The listing builds one solid part. Answer for the finished solid, in the listing's coordinates (mm). A direction names the side the tool comes from. Coordinates: 2 decimals unless noted, no trailing zeros. Order: outer loops, then holes, each group sorted by start corner. A loop starts at its lowest first (then second) coordinate and runs counter-clockwise, first axis right, second up. Notation, with made-up numbers: (9.5, 9.5) - (61.5, 9.5) arc R16 cw to (61.5, 37.5) - close; hole circle Ø2 at (74, 13). An arc over 180 degrees is marked (long way). Use a Markdown table: item, result. Add a question column.
Item 1: The part is cut by section C-C, the plane y = 3. Give the vertices of the cut face in (x, z).
Item 2: For faces 1 (the cylindrical face through (-17.572, 8.458, -3.902)), 2 (the flat face through (34, -20, 0)), determine the directions among +Z, -Z, +X, -X, +Y, -Y from which every point of the face is accessible in a straight line to the end or side of a thin tool.
Item 3: The part is cut by section D-D, the plane y = -6.5. Give the vertices of the cut face in (x, z), then the cut area to 3 significant figures.
Item 4: The part is cut by section A-A, the plane z = 0. Give the vertices of the cut face in (x, y), then the cut area to 3 significant figures.
Item 5: The part is cut by section B-B, the plane x = 0. Give the vertices of the cut face in (y, z).
Item 6: Flat-ended cylindrical pins translate along their axes: P1, Ø5, axis at y = -13, z = -0.5, coming from the +X side; P2, Ø12, axis at y = -0.5, z = 13.5, coming from the -X side; P3, Ø10, axis at x = -1, z = -2.5, coming from the +Y side; P4, Ø3, axis at y = 8.5, z = -5.5, coming from the +X side. Find the tip coordinate at first contact, or state that the pin passes through.
Item 7: Find the intervals of material crossed by line 1 along X through (y, z) = (4, 0); line 2 along X through (y, z) = (-5.75, 0); line 3 along Y through (x, z) = (30, 8), in increasing order.
from build123d import *

# Parameters (mm, degrees)
SKETCH1_R           = 18
BOSS_EXTRUDE1_DEPTH = 14
SKETCH2_R           = 3.25
BOSS_EXTRUDE2_DEPTH = 6
SKETCH3_R           = 10
SKETCH3_R_2         = 3.25
BOSS_EXTRUDE3_DEPTH = 20
CUT_EXTRUDE1_REACH  = 63.514
SKETCH4_R           = 10.75


with BuildPart() as part:
    # Sketch1 → Boss-Extrude1 (new body)
    with BuildSketch(Plane(origin=(0, 0, 0), x_dir=(1, 0, 0), z_dir=(0, 1, 0))):
        with Locations(Location((0, 0, 0), (0, 0, 270))):
            Circle(SKETCH1_R)
    extrude(amount=BOSS_EXTRUDE1_DEPTH)

    # Sketch2 → Boss-Extrude2 (add)
    with BuildSketch(Plane.XZ):
        with BuildLine():
            Line((40.105263158, 9.775881906), (3.789473684, 17.59658743))
            ThreePointArc((3.789473684, 17.59658743), (14.003758894, 11.309055524), (18, 0))
            ThreePointArc((18, 0), (14.003758894, -11.309055524), (3.789473684, -17.59658743))
            Line((3.789473684, -17.59658743), (40.105263158, -9.775881906))
            ThreePointArc((40.105263158, -9.775881906), (48, 0), (40.105263158, 9.775881906))
        make_face()
        with Locations(Location((38, 0, 0), (0, 0, 270))):
            Circle(SKETCH2_R, mode=Mode.SUBTRACT)
    extrude(amount=-BOSS_EXTRUDE2_DEPTH)

    # Sketch3 → Boss-Extrude3 (add)
    with BuildSketch(Plane.XZ):
        with Locations(Location((38, 0, 0), (0, 0, 270))):
            Circle(SKETCH3_R)
        with Locations(Location((38, 0, 0), (0, 0, 270))):
            Circle(SKETCH3_R_2, mode=Mode.SUBTRACT)
    extrude(amount=BOSS_EXTRUDE3_DEPTH)

    # Sketch4 → Cut-Extrude1 (cut, up to next)
    with BuildSketch(Plane(origin=(0, 14, 0), x_dir=(1, 0, 0), z_dir=(0, 1, 0)), mode=Mode.PRIVATE) as cut_extrude1_sk1:
        with Locations(Location((0, 0, 0), (0, 0, 270))):
            Circle(SKETCH4_R)
    cut_extrude1_tool1 = extrude(cut_extrude1_sk1.sketch, amount=-CUT_EXTRUDE1_REACH, mode=Mode.PRIVATE) & part.part
    add(cut_extrude1_tool1.solids().sort_by_distance((0, 14, 0))[0], mode=Mode.SUBTRACT)


solid = part.part
Solution:
| question | item | result |
|---|---|---|
| 1 | outline | (3.79, -17.6) - (40.11, -9.78) arc R10 ccw to (40.11, 9.78) - (3.79, 17.6) arc R18 ccw (long way) to start; hole circle Ø21.5 at (0, 0); hole circle Ø6.5 at (38, 0) |
| 2 | face 1 | +Y |
| 2 | face 2 | +Z, -Z, +X, -X, -Y |
| 3 | outline | circle Ø20 at (38, 0); hole circle Ø6.5 at (38, 0) |
| 3 | area | 281 mm2 |
| 4 | outline | (-18, 0) - (-10.75, 0) - (-10.75, 14) - (-18, 14) - close; (10.75, 0) - (28, 0) - (28, -20) - (34.75, -20) - (34.75, 6) - (18, 6) - (18, 14) - (10.75, 14) - close; (41.25, -20) - (48, -20) - (48, 6) - (41.25, 6) - close |
| 4 | area | 614 mm2 |
| 5 | outline | (0, -18) - (14, -18) - (14, -10.75) - (0, -10.75) - close; (0, 10.75) - (14, 10.75) - (14, 18) - (0, 18) - close |
| 6 | P1 | stops at x = 48 |
| 6 | P2 | stops at x = -16.35 |
| 6 | P3 | passes through |
| 6 | P4 | stops at x = 17.55 |
| 7 | line 1 | x = -18 to -10.75, 10.75 to 34.75, 41.25 to 48 |
| 7 | line 2 | x = 28 to 34.75, 41.25 to 48 |
| 7 | line 3 | y = 0 to 6 |
